Autodesk Inventor part; units mm, degrees
ref_plane "YZ Plane" through (0, 0, 0) normal (1, 0, 0) x (0, 1, 0)
ref_plane "XZ Plane" through (0, 0, 0) normal (0, 1, 0) x (-1, 0, 0)
ref_plane "XY Plane" through (0, 0, 0) normal (0, 0, 1) x (1, 0, 0)
sketch "Esquisse1" plane through (0, 0, 0) normal (0, 1, 0) x (-1, 0, 0)
  circle A0 centre (0, 0) radius 45.305
  circle A1 centre (0, 0) radius 47.7
  dimension "d0" = 90.61
  dimension "d1" = 95.4
extrude "Extrusion1" add sketch "Esquisse1" along normal blind 185
extrude "Extrusion2" add sketch "Esquisse1" along normal blind 2.5 contours A0
fillet "Congé1" radius 2 2 edges at (45.305, 2.5, 0) (47.7, 0, 0)
properties part number "Bocal"
Input: part model. Units: mm. Frame: model coordinates. A direction names the side the tool comes from. Coordinates: 2 decimals unless noted, no trailing zeros. Loops run counter-clockwise (first coordinate to the right, second up) from the corner with the lowest first, then second, coordinate; pieces in that order, holes last.
Q1. Draft query along Z for faces 3 (the face through (-45.497, 92.219, -14.328)), 4 (the face through (1, 2.5, 1)), 5 (the face through (1, 0, 1)). Return one class per face: +Z half, -Z half, draft (parallel to the pull), parting line (faces both ways), or undercut.
Q2. Material intervals for line 1 (Y direction, x = 20.5, z = -24.5); line 2 (Z direction, x = 0, y = 113) (3 decimals); line 3 (Z direction, x = -13, y = 79), sorted ascending.
Q3. Cut plane C-C (y = 118.5). Output: boundary loops of the cut face in (x, z) (3 decimals).
Q4. Set-up query: faces 1 (the face through (-42.2, 185, -17.4)), 2 (the face through (9.821, 93.486, 44.228)). Return all of +Z, -Z, +X, -X, +Y, -Y with unobstructed straight access to the full face (end or side cutting, diameter ignored); none if empty.
Q5. Cut plane A-A (x = 0). Output: boundary loops of the cut face in (y, z) (3 decimals).
Q6. Cut plane B-B (z = 0). Output: boundary loops of the cut face in (x, y) (3 decimals), then the cut area to 3 significant figures.
Q7. Contact query for flat-ended pins moving along their axis: pin 1 (5 mm diameter, centred on x = 13, y = 72, fed in from -Z); pin 2 (4 mm diameter, centred on x = -20, y = 57.5, fed in from +Z); pin 3 (6 mm diameter, centred on x = -28, z = 14, fed in from +Y). Output: stop coordinate, or through.
Working result:
1. face 3: parting line
1. face 4: undercut
1. face 5: draft
2. line 1: y = 0 to 2.5
2. line 2: z = -47.7 to -45.305, 45.305 to 47.7
2. line 3: z = -45.89 to -43.4, 43.4 to 45.89
3. outline: circle Ø95.4 at (0, 0); hole circle Ø90.61 at (0, 0)
4. face 1: +Z, -Z, +X, -X, +Y
4. face 2: +Y
5. outline: (0, -45.7) arc R2 ccw to (2, -47.7) - (185, -47.7) - (185, -45.305) - (4.5, -45.305) arc R2 cw to (2.5, -43.305) - (2.5, 43.305) arc R2 cw to (4.5, 45.305) - (185, 45.305) - (185, 47.7) - (2, 47.7) arc R2 ccw to (0, 45.7) - close
6. outline: (-47.7, 2) arc R2 ccw to (-45.7, 0) - (45.7, 0) arc R2 ccw to (47.7, 2) - (47.7, 185) - (45.305, 185) - (45.305, 4.5) arc R2 cw to (43.305, 2.5) - (-43.305, 2.5) arc R2 cw to (-45.305, 4.5) - (-45.305, 185) - (-47.7, 185) - close
6. area: 1,110 mm2
7. pin 1: stops at z = -46.53
7. pin 2: stops at z = 44.17
7. pin 3: stops at y = 2.5
